Can you work these out from the drawing? Everything is in mm from the part's minimum corner. A direction names the side the tool comes from. Give positions to 0.01 mm unless a question says otherwise; leave off trailing zeros. Loops run counter-clockwise (first coordinate to the right, second up) from the corner with the lowest first, then second, coordinate; pieces in that order, holes last. Notation, with made-up numbers: (-38, 24.5) -> (-20, 24.5) arc R10 ccw to (-20, 33.5) -> close; hole circle Ø3 at (70.25, 13). An arc over 180 degrees is marked (long way). Write item = value, one per line. Start each with the question number.
1) I'm going to push flat-ended pins straight in: pin 1 Ø6 at (y, z) = (26.5, 11.5) entering from -X; pin 2 Ø2 at (x, z) = (10.5, 16) entering from +Y. Where does each tip first touch, or does it pass through?
2) If we mould it in two halves opening along Z, with no side actions, what happens to the marked faces 1, 2 and 3? For each: +Z half, -Z half, draft (parallel to the pull), parting line (faces both ways), or undercut.
3) I want a section at B-B (z = 14). List the corners of the cut face in (x, y) for me.
4) I want a section at A-A (y = 39). List the corners of the cut face in (x, z) for me.
5) I need wall thicknesses on probe 1 along Z at (x, y) = (25, 35); probe 2 along Y at (x, z) = (79, 28); probe 3 along X at (y, z) = (4, 29.5). Which ranges of each line are inside material? Lowest first, please. Write a range as from..to.
6) I want a section at D-D (z = 25). List the corners of the cut face in (x, y) for me, and give its area (3 significant figures).
7) I want a section at C-C (y = 34). List the corners of the cut face in (x, z) for me.
8) On a 3-axis mill with a long thin cutter (end or side, diameter ignored), from which of +Z, -Z, +X, -X, +Y, -Y can I reach the whole of each face in a straight line? I mean the marked faces 4 and 5. Say none if no direction works.
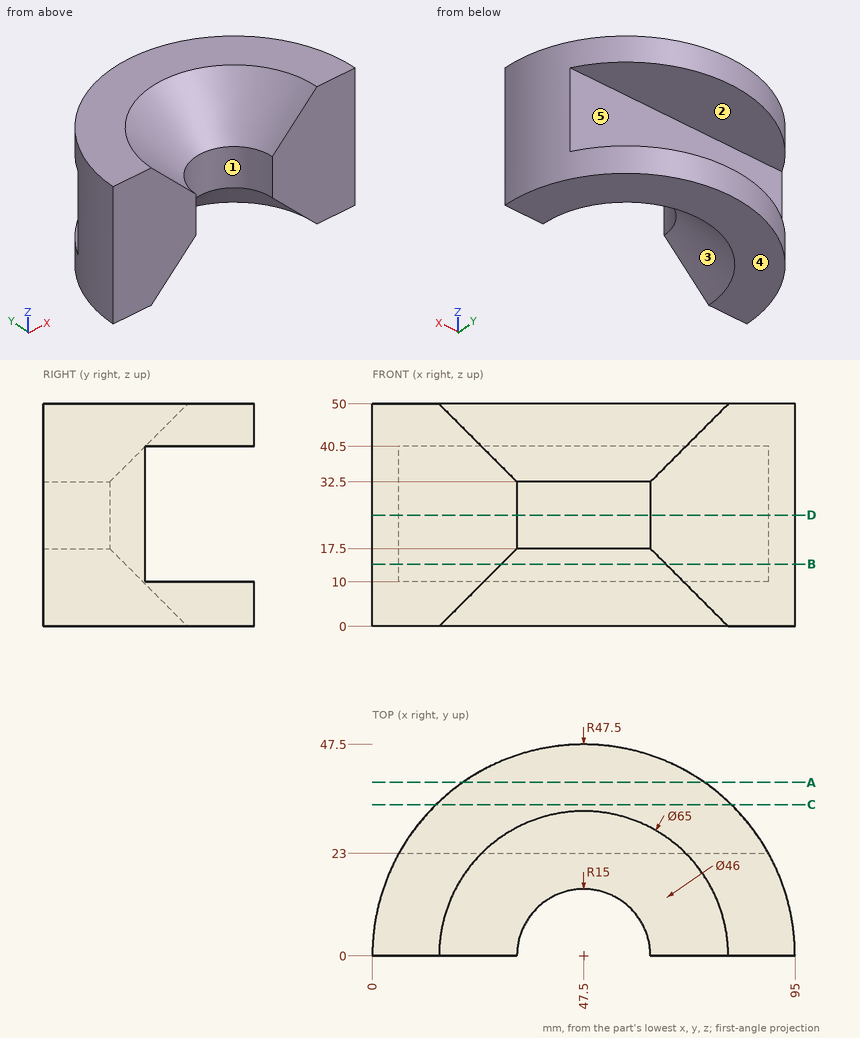
Answer list:
q1.pin_1 = 6.45
q1.pin_2 = 23
q2.face_1 = draft
q2.face_2 = undercut
q2.face_3 = -Z half
q3.outline = (0, 0) -> (29, 0) arc R18.5 cw to (66, 0) -> (95, 0) arc R47.5 ccw to (89.06, 23) -> (5.94, 23) arc R47.5 ccw to start
q4.outline = (20.38, 0) -> (74.62, 0) -> (74.62, 10) -> (20.38, 10) -> close; (20.38, 40.5) -> (74.62, 40.5) -> (74.62, 50) -> (20.38, 50) -> close
q5.probe_1 = 0..10, 40.5..50
q5.probe_2 = 0..23
q5.probe_3 = 0.17..33.04, 61.96..94.83
q6.outline = (0, 0) -> (32.5, 0) arc R15 cw to (62.5, 0) -> (95, 0) arc R47.5 ccw to (89.06, 23) -> (5.94, 23) arc R47.5 ccw to start
q6.area = 1,740 mm^2
q7.outline = (14.33, 0) -> (80.67, 0) -> (80.67, 10) -> (14.33, 10) -> close; (14.33, 40.5) -> (80.67, 40.5) -> (80.67, 50) -> (14.33, 50) -> close
q8.face_4 = -Z, +X, -X, +Y, -Y
q8.face_5 = +X, -X, +Y
